Verification items for the finished model (mm, model axes). Face numbers are marked on the shaded views. Give positions to 0.01 mm unless a question says otherwise; leave off trailing zeros. Order: outer loops, then holes, each group sorted by start corner. A loop starts at its lowest first (then second) coordinate and runs counter-clockwise, first axis right, second up. Notation, with made-up numbers: (-27.5, 89.25) -> (-12.5, 89.25) arc R18 ccw to (-12.5, 95.25) -> close; hole circle Ø8 at (-15, 77). An arc over 180 degrees is marked (long way). Return JSON: item names as keys, results as strings. Group by question number.
(1) Release check for a two-part mould opening along X. For the marked faces 1, 2 and 3 record: pulls with the +X half, pulls with the -X half, needs draft (parallel to the pull), parting line crosses it, or undercut.
(2) Thickness scan on line 1 along Y through (x, z) = (22, -4); line 2 along X through (y, z) = (4.6, -3.5); line 3 along X through (y, z) = (4.4, -2.75). Record the ranges inside material, lowest first.
(3) Cross-section at B-B on x = 16.5. Enter the section's corners in (y, z), then the cut area to 3 significant figures.
(4) Depth check by flat-ended pin: pin 1 Ø1.8 at (x, z) = (12, -3.5) entering from +Y; pin 2 Ø1.5 at (x, y) = (19, 5) entering from -Z. Enter the tip coordinate at first touch or a pass-through.
(5) Cross-section at A-A on y = 4.8. Enter the section's corners in (x, z).
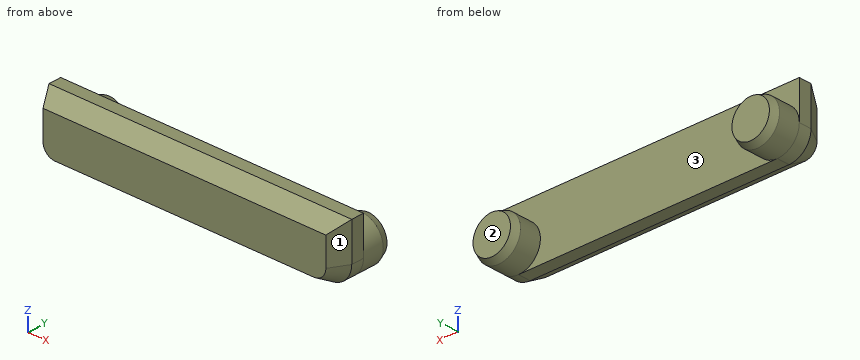
from build123d import *
from OCP.BRepFilletAPI import BRepFilletAPI_MakeChamfer
from build123d.topology import SkipClean

# Parameters (mm, degrees)
SKETCH1_W           = 30.4
SKETCH1_H           = 6
BOSS_EXTRUDE1_DEPTH = 3
SKETCH2_R           = 2.2
BOSS_EXTRUDE2_DEPTH = 2.9
CHAMFER1_SIZE       = 0.75
CHAMFER1_SIZE2      = 0.318356112
CUT_EXTRUDE1_START  = -3
CUT_EXTRUDE1_DEPTH  = 3
CHAMFER2_SIZE       = 1
CHAMFER2_SIZE2      = 1.732050808


with BuildPart() as part:
    # Sketch1 → Boss-Extrude1 (new body)
    with BuildSketch(Plane(origin=(0, 0, 0), x_dir=(1, 0, 0), z_dir=(0, 1, 0))):
        with Locations((15.2, 3)):
            Rectangle(SKETCH1_W, SKETCH1_H)
    extrude(amount=BOSS_EXTRUDE1_DEPTH)

    # Sketch2 → Boss-Extrude2 (add)
    with BuildSketch(Plane(origin=(0, 3, 0), x_dir=(1, 0, 0), z_dir=(0, 1, 0))):
        with Locations(Location((2.2, 3.8, 0), (0, 0, 90))):
            Circle(SKETCH2_R)
        with Locations(Location((28.2, 3.8, 0), (0, 0, 90))):
            Circle(SKETCH2_R)
    extrude(amount=BOSS_EXTRUDE2_DEPTH)

    # Chamfer1: one chamfer whose edges measure the first distance from different faces: ONE call of the kernel's chamfer builder (chamfer() names one face for all edges)
    chamfer1_edges_1 = [part.edges().sort_by_distance(p)[0] for p in [
        (2.2, 5.9, -1.6),
    ]]
    chamfer1_side_1 = [part.faces().sort_by_distance(p)[0] for p in [
        (2.2, 4.45, -1.6),
    ]]
    chamfer1_edges_2 = [part.edges().sort_by_distance(p)[0] for p in [
        (28.2, 5.9, -1.6),
    ]]
    chamfer1_side_2 = [part.faces().sort_by_distance(p)[0] for p in [
        (28.2, 4.45, -1.6),
    ]]
    chamfer1 = BRepFilletAPI_MakeChamfer(part.part.solid().wrapped)
    for e in chamfer1_edges_1:
        chamfer1.Add(CHAMFER1_SIZE, CHAMFER1_SIZE2, e.wrapped, chamfer1_side_1[0].wrapped)  # the first distance lies on this face
    for e in chamfer1_edges_2:
        chamfer1.Add(CHAMFER1_SIZE, CHAMFER1_SIZE2, e.wrapped, chamfer1_side_2[0].wrapped)  # the first distance lies on this face
    add(Compound.cast(chamfer1.Shape()), mode=Mode.REPLACE)

    # Sketch3 → Cut-Extrude1 (cut)
    with SkipClean():  # the faces are left unmerged after this step: merging them gives an invalid solid
        with BuildSketch(Plane(origin=(0, 3, 0), x_dir=(1, 0, 0), z_dir=(0, 1, 0)).offset(CUT_EXTRUDE1_START)):
            with BuildLine():
                Line((30.4, 3.8), (30.4, 6))
                Line((30.4, 6), (28.2, 6))
                ThreePointArc((28.2, 6), (29.755634919, 5.355634919), (30.4, 3.8))
            make_face()
            with BuildLine():
                Line((2.2, 6), (0, 6))
                Line((0, 6), (0, 3.8))
                ThreePointArc((0, 3.8), (0.644365081, 5.355634919), (2.2, 6))
            make_face()
        extrude(amount=CUT_EXTRUDE1_DEPTH, mode=Mode.SUBTRACT)

    # Chamfer2
    chamfer2_edges = [part.edges().sort_by_distance(p)[0] for p in [
        (0, 0, -1.9),
        (15.2, 0, -6),
        (29.755634919, 0, -5.355634919),
        (0.644365081, 0, -5.355634919),
        (30.4, 0, -1.9),
        (15.2, 0, 0),
    ]]
    chamfer2_side = [part.faces().sort_by_distance(p)[0] for p in [
        (15.2, 0, -2.971100636),
    ]]
    chamfer(chamfer2_edges, length=CHAMFER2_SIZE, length2=CHAMFER2_SIZE2, reference=chamfer2_side[0])


solid = part.part
Verdict:
{
 "1": {"face 1": "pulls with the +X half", "face 2": "needs draft", "face 3": "undercut"},
 "2": {"line 1": "0 to 3", "line 2": "0.02 to 4.38, 26.02 to 30.38", "line 3": "0.27 to 4.13, 26.27 to 30.13"},
 "3": {"outline": "(0, -5) -> (1.73, -6) -> (3, -6) -> (3, 0) -> (1.73, 0) -> (0, -1) -> close", "area": "16.3 mm²"},
 "4": {"pin 1": "y = 3", "pin 2": "through"},
 "5": {"outline": "circle Ø4.4 at (2.2, -3.8); circle Ø4.4 at (28.2, -3.8)"}
}
